Can you work these out from the drawing? Everything is in mm from the part's minimum corner. A direction names the side the tool comes from. Give positions to 0.01 mm unless a question says otherwise; leave off trailing zeros. Write each loop counter-clockwise with the first axis right and the second up, starting at its lowest first coordinate (ties: lowest second). Pieces come first, ordered by that corner, then holes. Notation, with made-up numbers: (15, 71) - (65, 71) arc R34 ccw to (65, 105) - close; hole circle Ø8 at (-32, -9). An arc over 180 degrees is marked (long way). Write each question's results on one line, items separated by ' | '. Start each with the question number.
Item 1: Suppose I cut it at D-D on x = 27.5. List the corners of the cut face in (y, z) for me (3 decimals), then the cut area to 3 significant figures.
Item 2: Please list where these lines run through material, in increasing order: line 1 along Z through (x, y) = (2.3, 12.7) (3 decimals); line 2 along X through (y, z) = (18.5, 69) (3 decimals); line 3 along Y through (x, z) = (0.85, 69.85) (3 decimals).
Item 3: Suppose I cut it at B-B on y = 12.5. List the corners of the cut face in (x, z) for me (3 decimals), then the cut area to 3 significant figures.
Item 4: Suppose I cut it at A-A on z = 44.45. List the corners of the cut face in (x, y) for me (3 decimals).
Item 5: Will these pins go through, and if not, where does the flat tip stop? P1, Ø1.5, axis at y = 35.5, z = 27, coming from the +X side (3 decimals); P2, Ø24, axis at x = 29.5, z = 40.5, coming from the -Y side (3 decimals).
Item 6: Which directions (+Z, -Z, +X, -X, +Y, -Y) give clear straight access to the entire face, cutting with the end or side of a thin tool? Please do the marked faces 1 and 2.
Item 7: Suppose I cut it at C-C on y = 19. List the corners of the cut face in (x, z) for me (3 decimals), then the cut area to 3 significant figures.
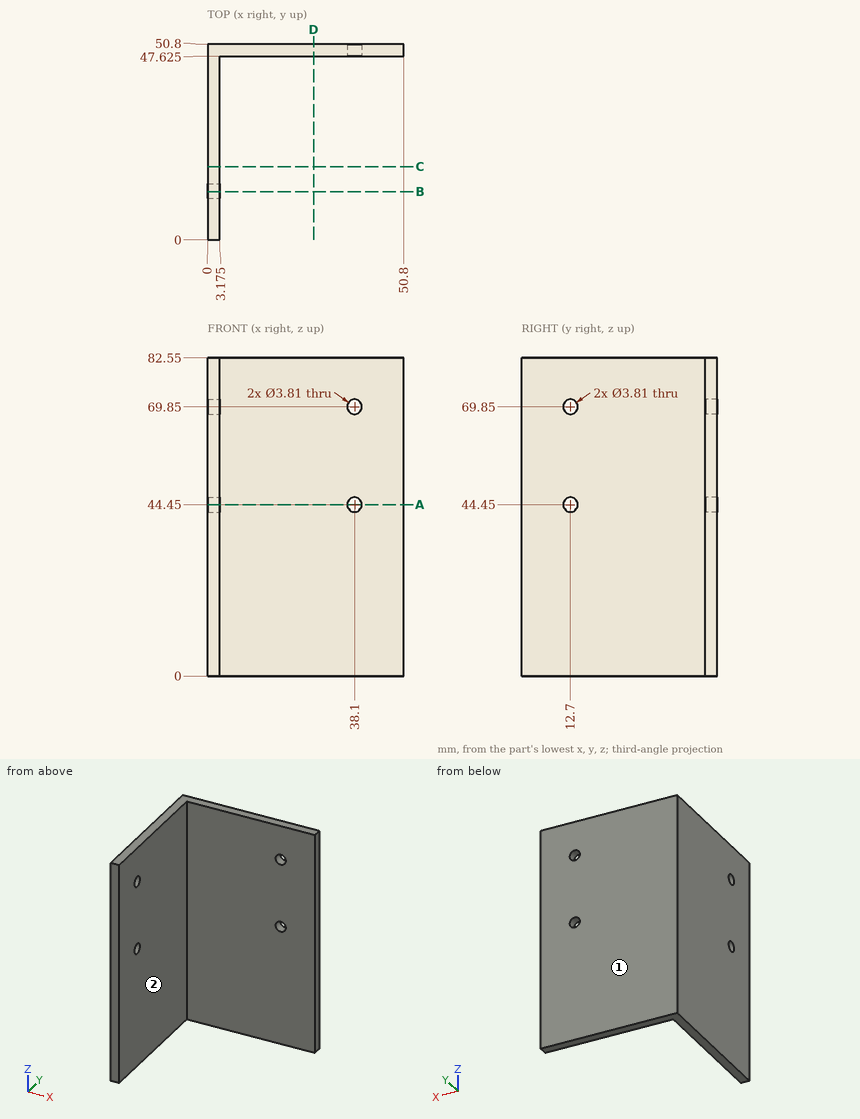
Checked values:
1) outline: (47.625, 0) - (50.8, 0) - (50.8, 82.55) - (47.625, 82.55) - close | area: 262 mm^2
2) line 1: z = 0 to 42.545, 46.355 to 67.945, 71.755 to 82.55 | line 2: x = 0 to 3.175 | line 3: y = 0 to 10.795, 14.605 to 50.8
3) outline: (0, 0) - (3.175, 0) - (3.175, 42.556) - (0, 42.556) - close; (0, 46.344) - (3.175, 46.344) - (3.175, 67.956) - (0, 67.956) - close; (0, 71.744) - (3.175, 71.744) - (3.175, 82.55) - (0, 82.55) - close | area: 238 mm^2
4) outline: (0, 0) - (3.175, 0) - (3.175, 10.795) - (0, 10.795) - close; (0, 14.605) - (3.175, 14.605) - (3.175, 47.625) - (36.195, 47.625) - (36.195, 50.8) - (0, 50.8) - close; (40.005, 47.625) - (50.8, 47.625) - (50.8, 50.8) - (40.005, 50.8) - close
5) P1: stops at x = 3.175 | P2: stops at y = 47.625
6) face 1: +Z, -Z, +X, -X, +Y | face 2: +Z, -Z, +X, -Y
7) outline: (0, 0) - (3.175, 0) - (3.175, 82.55) - (0, 82.55) - close | area: 262 mm^2
